from build123d import *

# Parameters (mm, degrees)
EXTRUDE_1_DEPTH     = 30
SKETCH_2_R          = 3.05
CUT_EXTRUDE_1_DEPTH = 30
SKETCH_3_R          = 3.05
CUT_EXTRUDE_2_DEPTH = 38


with BuildPart() as part:
    # 草图1 → 凸台-拉伸1 (new body)
    with BuildSketch(Plane.XY):
        Polygon((-15, 37.701761355), (-13, 37.701761355), (-13, -5.298238645), (13, -5.298238645), (13, 37.701761355), (15, 37.701761355), (15, -7.298238645), (-15, -7.298238645), align=None)
    extrude(amount=EXTRUDE_1_DEPTH)

    # 草图2 → 切除-拉伸1 (cut)
    with BuildSketch(Plane(origin=(0, 0, 0), x_dir=(1, 0, 0), z_dir=(0, 1, 0))):
        with Locations((0, -15)):
            Circle(SKETCH_2_R)
    extrude(amount=-CUT_EXTRUDE_1_DEPTH, mode=Mode.SUBTRACT)

    # 草图3 → 切除-拉伸2 (cut)
    with BuildSketch(Plane.ZY.offset(15)):
        with Locations((15, 27.701761355)):
            Circle(SKETCH_3_R)
    extrude(amount=-CUT_EXTRUDE_2_DEPTH, mode=Mode.SUBTRACT)


solid = part.part
Design review of the part built by this model. Coordinates are the model's own, in mm. A direction names the side the tool comes from. Round coordinates to 2 decimals unless told otherwise and drop trailing zeros. Loops run counter-clockwise (first coordinate to the right, second up) from the corner with the lowest first, then second, coordinate; pieces in that order, holes last. Notation, with made-up numbers: (13.5, -6.5) - (62.5, -6.5) arc R13 ccw to (62.5, 18.5) - close; hole circle Ø11 at (79, 20). An arc over 180 degrees is marked (long way). One line per question, with ' | ' between items.
1. For L1, parallel to Y at x = -13.45, z = 15; L2, parallel to X at y = 3, z = 11.5; L3, parallel to Z at x = 0, y = -6.8, list the stretches that pass through material, from the lowest coordinate up. Write a range as [from, to].
Results are:
L1: y = [-7.3, 24.65], [30.75, 37.7] | L2: x = [-15, -13], [13, 15] | L3: z = [0, 11.95], [18.05, 30]
2. We need section A-A, the plane x = 0. State the section outline as (y, z) points, and give its area (3 significant figures).
Results are:
outline: (-7.3, 0) - (-5.3, 0) - (-5.3, 11.95) - (-7.3, 11.95) - close; (-7.3, 18.05) - (-5.3, 18.05) - (-5.3, 30) - (-7.3, 30) - close | area: 47.8 mm²
3. For faces 5 (the face through (-13, 17, 15)), 6 (the face through (4, -7.298, 15)), list the 3-axis set-ups (+Z, -Z, +X, -X, +Y, -Y) from which the entire face can be reached by the end or side of a thin tool; tool diameter is ignored.
Results are:
face 5: +Z, -Z, +Y | face 6: +Z, -Z, +X, -X, -Y
4. Draft analysis for pull direction Y (two halves, no side actions). For faces 1 (the face through (0, -5.298, 11)), 2 (the face through (13.986, 24.996, 16.407)), 3 (the face through (-14.014, 24.996, 16.407)), 4 (the face through (13, 16, 15)), state which applies: released by +Y, released by -Y, zero draft, split by the parting line, or undercut.
Results are:
face 1: released by +Y | face 2: undercut | face 3: undercut | face 4: zero draft
5. We need section C-C, the plane y = 11. State the section outline as (x, z) points.
Results are:
outline: (-15, 0) - (-13, 0) - (-13, 30) - (-15, 30) - close; (13, 0) - (15, 0) - (15, 30) - (13, 30) - close
6. Clearance check with a flat-ended pin moving along its axis: P1, Ø8, axis at x = -5, z = 22.5, coming from the +Y side. State where the tip first meets the part, or that it passes through.
Results are:
P1: stops at y = -5.3
7. We need section D-D, the plane y = 26.5. State the section outline as (x, z) points.
Results are:
outline: (-15, 0) - (-13, 0) - (-13, 12.2) - (-15, 12.2) - close; (-15, 17.8) - (-13, 17.8) - (-13, 30) - (-15, 30) - close; (13, 0) - (15, 0) - (15, 12.2) - (13, 12.2) - close; (13, 17.8) - (15, 17.8) - (15, 30) - (13, 30) - close
8. We need section B-B, the plane z = 15. State the section outline as (x, y) points.
Results are:
outline: (-15, -7.3) - (-3.05, -7.3) - (-3.05, -5.3) - (-13, -5.3) - (-13, 24.65) - (-15, 24.65) - close; (-15, 30.75) - (-13, 30.75) - (-13, 37.7) - (-15, 37.7) - close; (3.05, -7.3) - (15, -7.3) - (15, 24.65) - (13, 24.65) - (13, -5.3) - (3.05, -5.3) - close; (13, 30.75) - (15, 30.75) - (15, 37.7) - (13, 37.7) - close
